from build123d import *

# Parameters (mm, degrees)
SKIZZE1_W                        = 139.5
SKIZZE1_H                        = 58
AUFSATZ_LINEAR_AUSTRAGEN1_DEPTH  = 28
SCHNITT_LINEAR_AUSTRAGEN2_DEPTH  = 30
VERRUNDUNG1_R                    = 8.5
SKIZZE5_W                        = 7.28
SKIZZE5_H                        = 30
SKIZZE5_W_2                      = 4
SKIZZE5_W_3                      = 4.15
SKIZZE5_W_4                      = 13.92
AUFSATZ_LINEAR_AUSTRAGEN2_DEPTH  = 4
VERRUNDUNG2_R                    = 5
AUFSATZ_LINEAR_AUSTRAGEN3_DEPTH  = 2
VERRUNDUNG3_R                    = 2
VERRUNDUNG4_R                    = 2
SKIZZE7_W                        = 139.5
SKIZZE7_H                        = 15
SCHNITT_LINEAR_AUSTRAGEN5_DEPTH  = 155.026783385
VERRUNDUNG5_R                    = 2
M2_5_GEWINDEBOHRUNG1_D           = 2.05
M2_5_GEWINDEBOHRUNG1_DEPTH       = 4.25
M2_5_GEWINDEBOHRUNG1_CSINK_D     = 2.55
M2_5_GEWINDEBOHRUNG1_CSINK_ANGLE = 90
M2_5_GEWINDEBOHRUNG1_TIP         = 0.615882135


with BuildPart() as part:
    # Skizze1 → Aufsatz-Linear austragen1 (new body)
    with BuildSketch(Plane(origin=(0, 0, 0), x_dir=(1, 0, 0), z_dir=(0, 1, 0))):
        with Locations((69.75, 29)):
            Rectangle(SKIZZE1_W, SKIZZE1_H)
    extrude(amount=AUFSATZ_LINEAR_AUSTRAGEN1_DEPTH)

    # Skizze4 → Schnitt-Linear austragen2 (cut)
    with BuildSketch(Plane(origin=(0, 0, -58), x_dir=(-1, 0, 0), z_dir=(0, 0, -1))):
        Polygon((-3.63, 0), (-80.58, 0), (-134.5, 0), (-134.5, 4), (-117.08, 4), (-117.08, 28), (-108.58, 28), (-100.08, 28), (-100.08, 4), (-89.08, 4), (-89.08, 28), (-72.08, 28), (-72.08, 4), (-60.93, 4), (-60.93, 28), (-43.93, 28), (-43.93, 4), (-32.9, 4), (-32.9, 28), (-15.9, 28), (-15.9, 4), (-5, 4), (-5, 0), align=None)
    extrude(amount=-SCHNITT_LINEAR_AUSTRAGEN2_DEPTH, mode=Mode.SUBTRACT)

    # Verrundung1
    verrundung1_edges = [part.edges().sort_by_distance(p)[0] for p in [
        (15.9, 16, -28),
        (32.9, 16, -28),
        (43.93, 16, -28),
        (60.93, 16, -28),
        (72.08, 16, -28),
        (89.08, 16, -28),
        (100.08, 16, -28),
        (117.08, 16, -28),
    ]]
    fillet(verrundung1_edges, radius=VERRUNDUNG1_R - 0.0001)  # a hair under: the kernel refuses the full size

    # Skizze5 → Aufsatz-Linear austragen2 (add)
    with BuildSketch(Plane.XZ.offset(-4)):
        with Locations((8.64, -43)):
            Rectangle(SKIZZE5_W, SKIZZE5_H)
        with Locations((94.58, -43)):
            Rectangle(SKIZZE5_W_2, SKIZZE5_H)
        with Locations((66.505, -43)):
            Rectangle(SKIZZE5_W_3, SKIZZE5_H)
        with Locations((38.355, -43)):
            Rectangle(SKIZZE5_W_3, SKIZZE5_H)
        with Locations((127.54, -43)):
            Rectangle(SKIZZE5_W_4, SKIZZE5_H)
    extrude(amount=AUFSATZ_LINEAR_AUSTRAGEN2_DEPTH)

    # Verrundung2
    verrundung2_edges = [part.edges().sort_by_distance(p)[0] for p in [
        (12.28, 2, -28),
        (96.58, 2, -28),
        (92.58, 2, -28),
        (68.58, 2, -28),
        (64.43, 2, -28),
        (120.58, 2, -28),
        (40.43, 2, -28),
        (36.28, 2, -28),
    ]]
    fillet(verrundung2_edges, radius=VERRUNDUNG2_R)

    # Skizze6 → Aufsatz-Linear austragen3 (add)
    with BuildSketch(Plane.XZ):
        with BuildLine():
            Line((139.5, -58), (134.5, -58))
            Line((134.5, -58), (134.5, -43))
            Line((134.5, -43), (135.978342998, -40.439434817))
            ThreePointArc((135.978342998, -40.439434817), (136.36732536, -39.500348322), (136.5, -38.492584381))
            Line((136.5, -38.492584381), (136.5, -28))
            ThreePointArc((136.5, -28), (135.035533906, -24.464466094), (131.5, -23))
            Line((131.5, -23), (129.007415619, -23))
            ThreePointArc((129.007415619, -23), (127.999651678, -23.13267464), (127.060565183, -23.521657002))
            Line((127.060565183, -23.521657002), (124.5, -25))
            Line((124.5, -25), (15, -25))
            Line((15, -25), (12.439434817, -23.521657002))
            ThreePointArc((12.439434817, -23.521657002), (11.500348322, -23.13267464), (10.492584381, -23))
            Line((10.492584381, -23), (8, -23))
            ThreePointArc((8, -23), (4.464466094, -24.464466094), (3, -28))
            Line((3, -28), (3, -38.492584381))
            ThreePointArc((3, -38.492584381), (3.13267464, -39.500348322), (3.521657002, -40.439434817))
            Line((3.521657002, -40.439434817), (5, -43))
            Line((5, -43), (5, -58))
            Line((5, -58), (0, -58))
            Line((0, -58), (0, 0))
            Line((0, 0), (139.5, 0))
            Line((139.5, 0), (139.5, -58))
        make_face()
    extrude(amount=AUFSATZ_LINEAR_AUSTRAGEN3_DEPTH)

    # Verrundung3
    verrundung3_edges = [part.edges().sort_by_distance(p)[0] for p in [
        (117.08, 16, -58),
        (100.08, 16, -58),
        (72.08, 16, -58),
        (43.93, 16, -58),
        (15.9, 16, -58),
        (32.9, 16, -58),
        (60.93, 16, -58),
        (89.08, 16, -58),
        (0, 13, -58),
        (139.5, 13, -58),
        (139.5, 13, 0),
        (0, 13, 0),
    ]]
    fillet(verrundung3_edges, radius=VERRUNDUNG3_R)

    # Verrundung4
    verrundung4_edges = [part.edges().sort_by_distance(p)[0] for p in [
        (12.28, 2, -58),
        (96.58, 2, -58),
        (92.58, 2, -58),
        (68.58, 2, -58),
        (64.43, 2, -58),
        (120.58, 2, -58),
        (40.43, 2, -58),
        (36.28, 2, -58),
        (5, -1, -58),
        (134.5, -1, -58),
    ]]
    fillet(verrundung4_edges, radius=VERRUNDUNG4_R - 0.0001)  # a hair under: the kernel refuses the full size

    # Skizze7 → Schnitt-Linear austragen5 (cut, through all)
    with BuildSketch(Plane(origin=(0, 28, 0), x_dir=(1, 0, 0), z_dir=(0, 1, 0))):
        with Locations((69.75, 7.5)):
            Rectangle(SKIZZE7_W, SKIZZE7_H)
    extrude(amount=-SCHNITT_LINEAR_AUSTRAGEN5_DEPTH, mode=Mode.SUBTRACT)

    # Verrundung5
    verrundung5_edges = [part.edges().sort_by_distance(p)[0] for p in [
        (139.5, 13, -15),
        (0, 13, -15),
    ]]
    fillet(verrundung5_edges, radius=VERRUNDUNG5_R)

    # M2.5 Gewindebohrung1
    with Locations(Plane(origin=(0, 0, 0), x_dir=(-1, 0, 0), z_dir=(0, -1, 0))):
        with Locations((-130.75, 32.3), (-8.75, 32.3)):
            CounterSinkHole(M2_5_GEWINDEBOHRUNG1_D / 2, M2_5_GEWINDEBOHRUNG1_CSINK_D / 2, depth=M2_5_GEWINDEBOHRUNG1_DEPTH, counter_sink_angle=M2_5_GEWINDEBOHRUNG1_CSINK_ANGLE)
            with Locations((0, 0, -(M2_5_GEWINDEBOHRUNG1_DEPTH + M2_5_GEWINDEBOHRUNG1_TIP / 2))):  # 118° drill point
                Cone(0, M2_5_GEWINDEBOHRUNG1_D / 2, M2_5_GEWINDEBOHRUNG1_TIP, mode=Mode.SUBTRACT)


solid = part.part
Source: CAD feature listing. Evaluate the final solid. Frame: model axes, mm. A direction names the side the tool comes from. Give positions to 0.01 mm unless a question says otherwise; leave off trailing zeros. Answer as a JSON object with one key per item and string values.
Q1. Mould query, pull axis Z, two halves, no side actions, for faces 1 (the face through (18.32, 15.83, -30.56)), 2 (the face through (135.07, -0.99, -24.5)), 3 (the face through (15, 4, -42)). Classes: +Z half, -Z half, draft (parallel to the pull), parting line (faces both ways), or undercut.
Geometry check:
{"face 1": "-Z half", "face 2": "undercut", "face 3": "draft"}
Q2. Cut plane A-A, the plane z = -51.5. Count the separate pieces of the cut face and the enclosed holes in it, then the cut area to 3 significant figures.
Geometry check:
{"separate pieces": "5", "enclosed holes": "0", "area": "1,910 mm^2"}
Q3. Ray query, line 1 along X through (y, z) = (18.75, -53); line 2 along Z through (x, y) = (130.75, 1.6) (3 decimals); line 3 along Z through (x, y) = (103, 1.75). Return the intervals inside material, ascending.
Geometry check:
{"line 1": "x = 0 to 15.9, 32.9 to 43.93, 60.93 to 72.08, 89.08 to 100.08, 117.08 to 139.5", "line 2": "z = -58 to -33.325, -31.275 to -15", "line 3": "z = -28 to -15"}
Q4. Contact query for flat-ended pins moving along their axis: P1, Ø6, axis at x = 69, z = -36.5, coming from the -Y side; P2, Ø2, axis at x = 130, y = -1.5, coming from the -Z side; P3, Ø0.6, axis at x = 62.5, y = -1, coming from the -Z side. Output: stop coordinate, or through.
Geometry check:
{"P1": "stops at y = 0", "P2": "stops at z = -23", "P3": "stops at z = -25"}
Q5. Access query for faces 4 (the face through (5, -1, -24)), 5 (the face through (52, 3, -28)), 6 (the face through (60.93, 16, -46)). Directions: +Z, -Z, +X, -X, +Y, -Y. A direction counts if a zero-diameter tool reaches every point of the face in a straight line with its end or side. Return the directions, or none.
Geometry check:
{"face 4": "-Y", "face 5": "-Z, -Y", "face 6": "-Z, +Y, -Y"}
